For this review, use the dimensioned drawing (mm, ordinates from the lowest corner) and the shaded views. A direction names the side the tool comes from. Coordinates: 2 decimals unless noted, no trailing zeros. Loops run counter-clockwise (first coordinate to the right, second up) from the corner with the lowest first, then second, coordinate; pieces in that order, holes last. Notation, with made-up numbers: M 12,71.25 L 44,71.25 A12 ccw 44,77.25 Z; hole C -1.5,1.5 d9. An arc over 180 degrees is marked long. Write item = value, one per line.
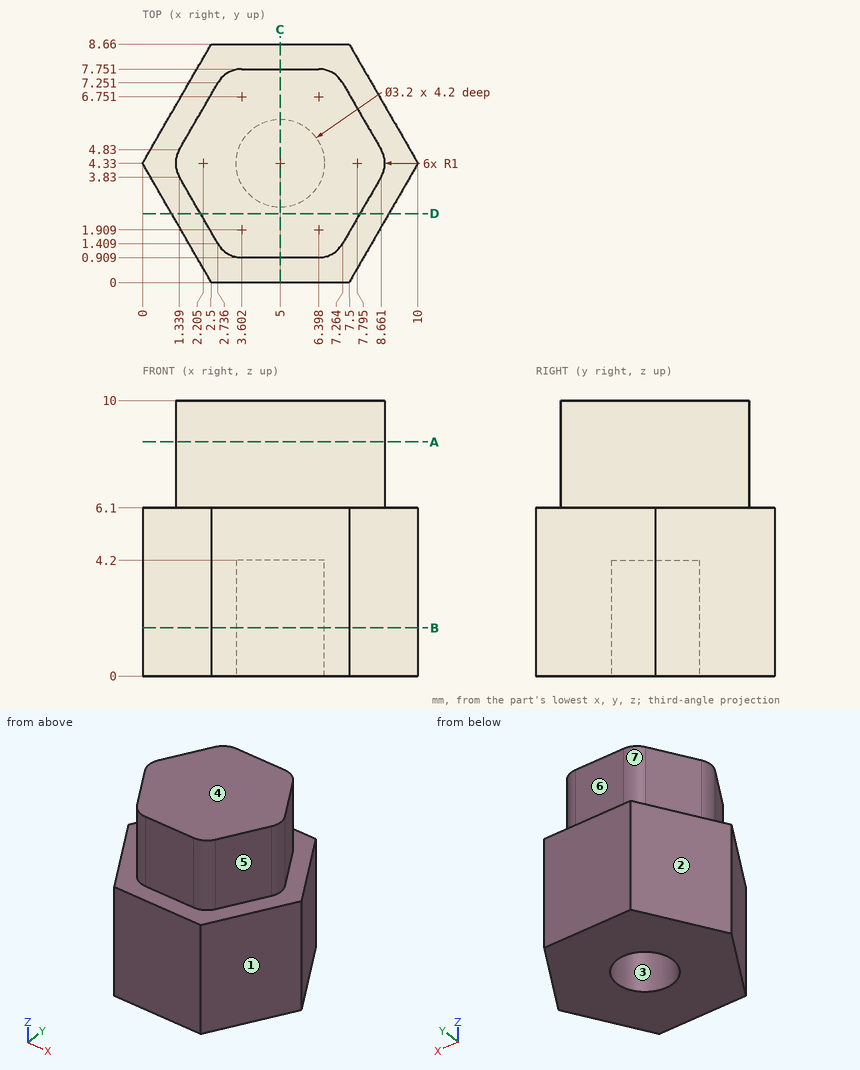
Q1. For line 1 along Y through (x, z) = (5, 2.05); line 2 along Z through (x, y) = (1, 5.75); line 3 along Y through (x, z) = (3.75, 8), list the stretches that pass through material, from the lowest coordinate up.
Solved:
line_1 = 0 to 2.73, 5.93 to 8.66
line_2 = 0 to 6.1
line_3 = 0.91 to 7.75
Q2. Add section B-B (z = 1.75). Write out the cut boundary in (x, y).
Solved:
outline = M 0,4.33 L 2.5,0 L 7.5,0 L 10,4.33 L 7.5,8.66 L 2.5,8.66 Z; hole C 5,4.33 d3.2
Q3. For pin 1 Ø0.8 at (x, z) = (5.5, 8) entering from +Y; pin 2 Ø1.4 at (x, z) = (5, 8) entering from -Y; pin 3 Ø1.5 at (x, z) = (1, 7.5) entering from -Y, all flat-tipped, find the tip position at first contact; note any pin that passes through.
Solved:
pin_1 = 7.75
pin_2 = 0.91
pin_3 = 3.12
Q4. Draft analysis for pull direction Y (two halves, no side actions). For the marked faces 1, 2, 3 and 4, state which applies: +Y half, -Y half, draft (parallel to the pull), parting line (faces both ways), or undercut.
Solved:
face_1 = -Y half
face_2 = +Y half
face_3 = undercut
face_4 = draft
Q5. Add section C-C (x = 5). Write out the cut boundary in (y, z).
Solved:
outline = M 0,0 L 2.73,0 L 2.73,4.2 L 5.93,4.2 L 5.93,0 L 8.66,0 L 8.66,6.1 L 7.75,6.1 L 7.75,10 L 0.91,10 L 0.91,6.1 L 0,6.1 Z
Q6. Add section D-D (y = 2.5). Write out the cut boundary in (x, z), and give its area (3 significant figures).
Solved:
outline = M 1.06,0 L 8.94,0 L 8.94,6.1 L 7.89,6.1 L 7.89,10 L 2.11,10 L 2.11,6.1 L 1.06,6.1 Z
area = 70.7 mm²
Q7. Add section A-A (z = 8.5). Write out the cut boundary in (x, y) (1 decimal).
Solved:
outline = M 1.3,3.8 L 2.7,1.4 A1 ccw 3.6,0.9 L 6.4,0.9 A1 ccw 7.3,1.4 L 8.7,3.8 A1 ccw 8.7,4.8 L 7.3,7.3 A1 ccw 6.4,7.8 L 3.6,7.8 A1 ccw 2.7,7.3 L 1.3,4.8 A1 ccw Z
Q8. Machinability: for the marked faces 5, 6 and 7, which of the approach directions +Z, -Z, +X, -X, +Y, -Y give a long, thin tool a straight path to every point of the face, cutting with its end or side? Answer none if there is none.
Solved:
face_5 = +Z, +X, -Y
face_6 = +Z, +X, -X, +Y
face_7 = +Z, -X, +Y
